```python
from build123d import *

# Parameters (mm, degrees)
SKETCH1_R           = 7
BOSS_EXTRUDE1_DEPTH = 11
SKETCH2_R           = 2.5
CUT_EXTRUDE1_DEPTH  = 6.5
SKETCH3_R           = 4
CUT_EXTRUDE2_DEPTH  = 6.5


with BuildPart() as part:
    # Sketch1 → Boss-Extrude1 (new, symmetric)
    with BuildSketch(Plane.XY):
        Circle(SKETCH1_R)
    extrude(amount=BOSS_EXTRUDE1_DEPTH, both=True)

    # Sketch2 → Cut-Extrude1 (cut)
    with BuildSketch(Plane.XY.offset(11)):
        Circle(SKETCH2_R)
    extrude(amount=-CUT_EXTRUDE1_DEPTH, mode=Mode.SUBTRACT)

    # Sketch3 → Cut-Extrude2 (cut)
    with BuildSketch(Plane(origin=(0, 0, -11), x_dir=(-1, 0, 0), z_dir=(0, 0, -1))):
        Circle(SKETCH3_R)
    extrude(amount=-CUT_EXTRUDE2_DEPTH, mode=Mode.SUBTRACT)


solid = part.part
```
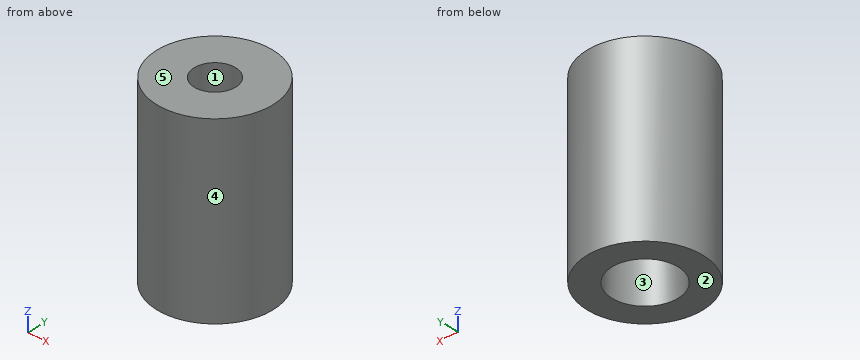
CAD build for the part. Positions are in the model's coordinates, mm. Face numbers are marked on the shaded views. A direction names the side the tool comes from. Round coordinates to 2 decimals unless told otherwise and drop trailing zeros. Write each loop counter-clockwise with the first axis right and the second up, starting at its lowest first coordinate (ties: lowest second). Pieces come first, ordered by that corner, then holes. Notation, with made-up numbers: (88.5, 32) - (106.5, 32) arc R23 ccw to (106.5, 67) - close; hole circle Ø3 at (76, 60.5). An arc over 180 degrees is marked (long way). Write item = value, one per line. Start each with the question number.
Q1. Band-saw the part on D-D (z = -2.75). Give the cut face in (x, y), then the cut area to 3 significant figures.
Q2. Which spindle directions (+Z, -Z, +X, -X, +Y, -Y) get a long thin tool onto all of the face, cutting with end or side? Do the marked faces 1 and 2. Say none if no direction does.
Q3. Band-saw the part on A-A (y = 0). Give the cut face in (x, z).
Q4. Drop flat-ended pins along their axis: pin 1 (4 mm diameter, centred on x = 1, y = -1, fed in from +Z); pin 2 (1.5 mm diameter, centred on y = 2.5, z = -3.5, fed in from +X); pin 3 (4 mm diameter, centred on y = -4.5, z = 8.5, fed in from +X); pin 4 (3 mm diameter, centred on y = -3.5, z = 3.5, fed in from +X). Give the stop position or say it passes through.
Q5. Band-saw the part on C-C (z = -6). Give the cut face in (x, y).
Q6. Probe L1, parallel to Y at x = 0, z = -6; L2, parallel to Y at x = 0, z = 7.25; L3, parallel to Z at x = 2, y = -3. List the from-to ranges inside material, lowest first. Write a range as from..to.
Q7. Mould opens along Y. For the marked faces 3, 4 and 5 say: pulls with the +Y half, pulls with the -Y half, needs draft (parallel to the pull), parting line crosses it, or undercut.
Answers below:
q1.outline = circle Ø14 at (0, 0)
q1.area = 154 mm2
q2.face_1 = +Z
q2.face_2 = -Z, +X, -X, +Y, -Y
q3.outline = (-7, -11) - (-4, -11) - (-4, -4.5) - (4, -4.5) - (4, -11) - (7, -11) - (7, 11) - (2.5, 11) - (2.5, 4.5) - (-2.5, 4.5) - (-2.5, 11) - (-7, 11) - close
q4.pin_1 = 11
q4.pin_2 = 6.78
q4.pin_3 = 6.54
q4.pin_4 = 6.71
q5.outline = circle Ø14 at (0, 0); hole circle Ø8 at (0, 0)
q6.L1 = -7..-4, 4..7
q6.L2 = -7..-2.5, 2.5..7
q6.L3 = -4.5..11
q7.face_3 = undercut
q7.face_4 = parting line crosses it
q7.face_5 = needs draft
